Input: part model. Units: mm. Frame: model coordinates. Face numbers are marked on the shaded views. Round coordinates to 2 decimals unless told otherwise and drop trailing zeros. Loops run counter-clockwise (first coordinate to the right, second up) from the corner with the lowest first, then second, coordinate; pieces in that order, holes last.
(1) Cut plane C-C, the plane x = 18.5. Output: boundary loops of the cut face in (y, z) (3 decimals), and give its area (3 significant figures).
(2) Cut plane A-A, the plane z = -7. Output: boundary loops of the cut face in (x, y) (1 decimal), and give its area (3 significant figures).
(3) First-contact query: pin 1 Ø3.5 at (x, y) = (-4.76, -4.78) entering from -Z; pin 2 Ø5 at (x, z) = (58, 3.5) entering from +Y. Flat tips, straight axial feed; report the tip coordinate or a pass-through.
(4) Draft query along Z for the marked faces 1, 2, 3 and 4. Return one class per face: released by +Z, released by -Z, zero draft, split by the parting line, or undercut.
(5) Line query: line 1 (X direction, y = -6.5, z = -7.5) (3 decimals); line 2 (X direction, y = -3.25, z = 1) (3 decimals); line 3 (Z direction, x = -50.5, y = -2.5). Output: solid intervals per line, ascending.
(6) Cut plane B-B, the plane x = 54.5. Output: boundary loops of the cut face in (y, z) (3 decimals), and give its area (3 significant figures).
from build123d import *

# Parameters (mm, degrees)
F0_R     = 6.35
F0_R_2   = 3.175
F1_DEPTH = 9.525
F3_D     = 4.0386
F3_DEPTH = 22.70125
F3_TIP   = 1.213317848
F5_D     = 4.0386
F5_DEPTH = 11.90625
F5_TIP   = 1.213317848
F7_D     = 4.0386
F7_DEPTH = 22.7076
F7_TIP   = 1.213317848


with BuildPart() as f1:
    # F0 (on Front) → F1 (new body)
    with BuildSketch(Plane.XZ):
        with BuildLine():
            Line((-3.175, 19.05), (-79.375, 19.05))
            Line((-79.375, 19.05), (-79.375, -19.05))
            Line((-79.375, -19.05), (79.375, -19.05))
            Line((79.375, -19.05), (79.375, 19.05))
            Line((79.375, 19.05), (74.6070611226, 19.05))
            ThreePointArc((74.6070611226, 19.05), (70.7998475457, 17.7820886237), (68.513014884, 14.4846849699))
            Line((68.513014884, 14.4846849699), (64.643, 1.27))
            Line((64.643, 1.27), (-3.175, 19.05))
        make_face()
        with Locations((-47.625, 9.525)):
            Circle(F0_R, mode=Mode.SUBTRACT)
        with Locations((73.7743, 13.97)):
            Circle(F0_R_2, mode=Mode.SUBTRACT)
    extrude(amount=F1_DEPTH)

    # F3
    with Locations(Plane(origin=(-79.375, 0, 0), x_dir=(0, -1, 0), z_dir=(-1, 0, 0))):
        with Locations((4.7625112989, 14.2875), (4.7751887011, -14.2875)):
            Hole(F3_D / 2, depth=F3_DEPTH)
            with Locations((0, 0, -(F3_DEPTH + F3_TIP / 2))):  # 118° drill point
                Cone(0, F3_D / 2, F3_TIP, mode=Mode.SUBTRACT)

    # F5
    with Locations(Plane.XY.offset(19.05)):
        with Locations((-47.625, -4.7498)):
            Hole(F5_D / 2, depth=F5_DEPTH)
            with Locations((0, 0, -(F5_DEPTH + F5_TIP / 2))):  # 118° drill point
                Cone(0, F5_D / 2, F5_TIP, mode=Mode.SUBTRACT)

    # F7
    with Locations(Plane(origin=(0, 0, -19.05), x_dir=(1, 0, 0), z_dir=(0, 0, -1))):
        with Locations((-38.1, 4.7625), (-4.7625, 4.7752), (28.575, 4.7752)):
            Hole(F7_D / 2, depth=F7_DEPTH)
            with Locations((0, 0, -(F7_DEPTH + F7_TIP / 2))):  # 118° drill point
                Cone(0, F7_D / 2, F7_TIP, mode=Mode.SUBTRACT)


solid = f1.part
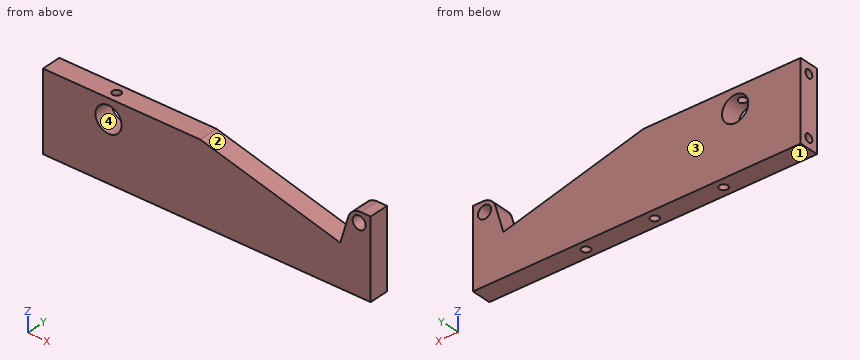
Reported:
1. outline: (-9.525, -19.05) - (0, -19.05) - (0, 13.367) - (-9.525, 13.367) - close
1. area: 309 mm2
2. outline: (-79.4, -9.5) - (79.4, -9.5) - (79.4, 0) - (-79.4, 0) - close; hole circle Ø4 at (-38.1, -4.8); hole circle Ø4 at (-4.8, -4.8); hole circle Ø4 at (28.6, -4.8)
2. area: 1,470 mm2
3. pin 1: stops at z = 3.82
3. pin 2: stops at y = 0
4. face 1: released by -Z
4. face 2: released by +Z
4. face 3: zero draft
4. face 4: undercut
5. line 1: x = -79.375 to -39.129, -37.071 to -5.813, -3.712 to 27.525, 29.625 to 79.375
5. line 2: x = -79.375 to -39.438, -36.762 to -6.086, -3.439 to 27.252, 29.898 to 79.375
5. line 3: z = -19.05 to 3.86, 15.19 to 19.05
6. outline: (-9.525, -19.05) - (0, -19.05) - (0, 3.929) - (-9.525, 3.929) - close
6. area: 219 mm2
